```python
from build123d import *

# Parameters (mm, degrees)
BOX002_W     = 10
BOX002_H     = 10
BOX002_DEPTH = 16
BOX001_W     = 14
BOX001_H     = 14
BOX001_DEPTH = 10
BOX_W        = 16
BOX_H        = 16
BOX_DEPTH    = 10


with BuildPart() as cube001:
    # Box002 → Box002 (new body)
    with BuildSketch(Plane(origin=(-5, -5, 0), x_dir=(1, 0, 0), z_dir=(0, 0, 1))):
        with Locations((5, 5)):
            Rectangle(BOX002_W, BOX002_H)
    extrude(amount=BOX002_DEPTH)


with BuildPart() as cubo:
    # Box001 → Box001 (new body)
    with BuildSketch(Plane(origin=(-7, -7, 10), x_dir=(1, 0, 0), z_dir=(0, 0, 1))):
        with Locations((7, 7)):
            Rectangle(BOX001_W, BOX001_H)
    extrude(amount=BOX001_DEPTH)


with BuildPart() as common:
    # Sphere → Sphere (revolve)
    with BuildSketch(Plane.XZ):
        with BuildLine():
            ThreePointArc((0, -20), (20, 0), (0, 20))
            Line((0, 20), (0, -20))
        make_face()
    revolve(axis=Axis((0, 0, 0), (0, 0, 1)))

    # Common: intersect Cubo
    add(cubo.part, mode=Mode.INTERSECT)


with BuildPart() as cut:
    # Box → Box (new body)
    with BuildSketch(Plane(origin=(-8, -8, 0), x_dir=(1, 0, 0), z_dir=(0, 0, 1))):
        with Locations((8, 8)):
            Rectangle(BOX_W, BOX_H)
    extrude(amount=BOX_DEPTH)

    # Fusion: union Common
    add(common.part)

    # Cut: cut Cube001
    add(cube001.part, mode=Mode.SUBTRACT)


solid = cut.part
```
Here's how the part is built. I have some questions about the finished solid (model axes, mm). A direction names the side the tool comes from. Give positions to 0.01 mm unless a question says otherwise; leave off trailing zeros. Loops run counter-clockwise (first coordinate to the right, second up) from the corner with the lowest first, then second, coordinate; pieces in that order, holes last. Notation, with made-up numbers: M 58,-17 L 85,-17 A21 cw 85,0 Z; hole C 0,60 d2. An arc over 180 degrees is marked long. Return JSON: item names as keys, results as strings.
Item 1: Imagine slicing it at A-A on z = 13.25. List the corners of the cut face in (x, y) for me.
A:
{"outline": "M -7,-7 L 7,-7 L 7,7 L -7,7 Z; hole M -5,-5 L 5,-5 L 5,5 L -5,5 Z"}
Item 2: Imagine slicing it at C-C on x = 1.75. List the corners of the cut face in (y, z) for me.
A:
{"outline": "M -8,0 L -5,0 L -5,16 L 5,16 L 5,0 L 8,0 L 8,10 L 7,10 L 7,18.65 A19.92 ccw -7,18.65 L -7,10 L -8,10 Z"}
Item 3: Please list where these lines run through material, in increasing order: line 1 (Y direction, x = 4.75, z = 1.75); line 2 (Y direction, x = -4, z = 15.25).
A:
{"line 1": "y = -8 to -5, 5 to 8", "line 2": "y = -7 to -5, 5 to 7"}
Item 4: I'm going to push flat-ended pins straight in: pin 1 Ø6 at (x, z) = (4, 17.5) entering from +Y; pin 2 Ø6 at (y, z) = (6, 14.5) entering from -X. Where does each tip first touch, or does it pass through?
A:
{"pin 1": "stops at y = 7", "pin 2": "stops at x = -7"}
Item 5: Thinking about a two-plate mould opening in Y: for faces 1 (the flat face through (0, -7, 14)), 2 (the flat face through (-7.15, 0.04, 10)), 3 (the flat face through (0, -5, 8)), which applies, released by +Y, released by -Y, zero draft, split by the parting line, or undercut?
A:
{"face 1": "released by -Y", "face 2": "zero draft", "face 3": "undercut"}
Item 6: On a 3-axis mill with a long thin cutter (end or side, diameter ignored), from which of +Z, -Z, +X, -X, +Y, -Y can I reach the whole of each face in a straight line? I mean faces 4 (the flat face through (-7, 0, 14)), 5 (the flat face through (5, 0, 8)), 6 (the flat face through (0, 7, 14)), 7 (the flat face through (7, 0, 14)). Say none if no direction works.
A:
{"face 4": "+Z, -X, +Y, -Y", "face 5": "-Z", "face 6": "+Z, +X, -X, +Y", "face 7": "+Z, +X, +Y, -Y"}
Item 7: Imagine slicing it at B-B on y = -3.5. List the corners of the cut face in (x, z) for me, then the cut area to 3 significant figures.
A:
{"outline": "M -8,0 L -5,0 L -5,16 L 5,16 L 5,0 L 8,0 L 8,10 L 7,10 L 7,18.41 A19.69 ccw -7,18.41 L -7,10 L -8,10 Z", "area": "130 mm^2"}
Item 8: Imagine slicing it at D-D on z = 1.75. List the corners of the cut face in (x, y) for me, then the cut area to 3 significant figures.
A:
{"outline": "M -8,-8 L 8,-8 L 8,8 L -8,8 Z; hole M -5,-5 L 5,-5 L 5,5 L -5,5 Z", "area": "156 mm^2"}
